Job drawing, mm, ordinate dimensions from the low corner. One solid piece. A direction names the side the tool comes from. Round coordinates to 2 decimals unless told otherwise and drop trailing zeros. Loops run counter-clockwise (first coordinate to the right, second up) from the corner with the lowest first, then second, coordinate; pieces in that order, holes last.
1) Band-saw the part on C-C, the plane z = 11. Write the cut outline in (x, y), then the cut area to 3 significant figures.
2) Drop flat-ended pins along their axis: P1, Ø19.5, axis at y = 24, z = 7, coming from the -X side; P2, Ø1.8, axis at x = 49.55, z = 29.81, coming from the +Y side; P3, Ø5.5, axis at y = 19.5, z = 8.5, coming from the +X side; P4, Ø5.5, axis at x = 5.5, y = 1.5, coming from the -Z side. Give the stop position or say it passes through.
3) Band-saw the part on D-D, the plane x = 23. Write the cut outline in (y, z) (1 decimal), then the cut area to 3 significant figures.
4) 3-axis set-ups, long thin cutter, end or side, ignore diameter. For the marked faces 4, 5 and 6: which of +Z, -Z, +X, -X, +Y, -Y reach the whole face in a straight line?
5) Band-saw the part on A-A, the plane x = 16. Write the cut outline in (y, z) (1 decimal), then the cut area to 3 significant figures.
6) Mould opens along X. For the marked faces 1, 2 and 3 say: +X half, -X half, draft (parallel to the pull), parting line (faces both ways), or undercut.
7) Band-saw the part on B-B, the plane y = 25. Write the cut outline in (x, z).
8) Probe line 1 (Z direction, x = 20, y = 23.5); line 2 (Y direction, x = 19, z = 28.5); line 3 (Z direction, x = 26.5, y = 4.5) (1 decimal). List the from-to ranges inside material, lowest first.
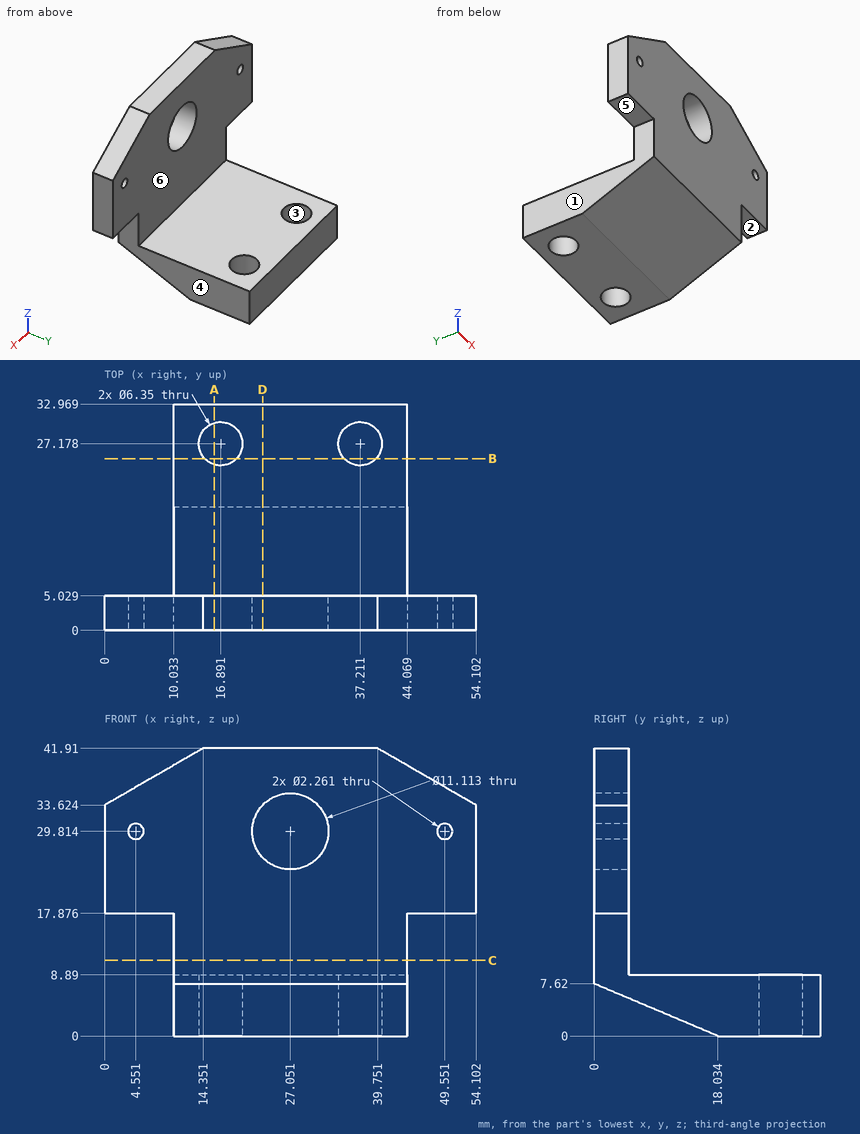
Reported:
1. outline: (10.03, 0) - (44.07, 0) - (44.07, 5.03) - (10.03, 5.03) - close
1. area: 171 mm2
2. P1: stops at x = 10.03
2. P2: passes through
2. P3: stops at x = 44.07
2. P4: stops at z = 17.88
3. outline: (0, 7.6) - (18, 0) - (33, 0) - (33, 8.9) - (5, 8.9) - (5, 26) - (0, 26) - close; (0, 33.6) - (5, 33.6) - (5, 41.9) - (0, 41.9) - close
3. area: 352 mm2
4. face 4: -Z, +X, +Y, -Y
4. face 5: -Z, -X, +Y, -Y
4. face 6: +Z, +X, -X, +Y
5. outline: (0, 7.6) - (18, 0) - (24.1, 0) - (24.1, 8.9) - (5, 8.9) - (5, 41.9) - (0, 41.9) - close; (30.2, 0) - (33, 0) - (33, 8.9) - (30.2, 8.9) - close
5. area: 336 mm2
6. face 1: -X half
6. face 2: draft
6. face 3: undercut
7. outline: (10.03, 0) - (14.58, 0) - (14.58, 8.89) - (10.03, 8.89) - close; (19.2, 0) - (34.9, 0) - (34.9, 8.89) - (19.2, 8.89) - close; (39.52, 0) - (44.07, 0) - (44.07, 8.89) - (39.52, 8.89) - close
8. line 1: z = 0 to 8.89
8. line 2: y = 0 to 5.03
8. line 3: z = 5.7 to 24.3, 35.3 to 41.9
